from build123d import *

# Parameters (mm, degrees)
ESBO_O1_W                                            = 100
ESBO_O1_H                                            = 40
BASEPLATE_DEPTH                                      = 10
VERTBOSS_DEPTH                                       = 10
ESBO_O3_W                                            = 39.225392784
ESBO_O3_H                                            = 3
BOTTOMSLOT_DEPTH                                     = 121.933866224
REBAIXO_PARA_PARAFUSO_DE_CABE_A_SEXTAVAD_D           = 9
REBAIXO_PARA_PARAFUSO_DE_CABE_A_SEXTAVAD_CBORE_D     = 18.01
REBAIXO_PARA_PARAFUSO_DE_CABE_A_SEXTAVAD_CBORE_DEPTH = 5.68
FILETE1_R                                            = 8
FILETE2_R                                            = 3
FURO_DE_DI_METRO_7_0_7_2_D                           = 7


with BuildPart() as part:
    # Esboço1 → BasePlate (new body)
    with BuildSketch(Plane(origin=(0, 0, 0), x_dir=(1, 0, 0), z_dir=(0, 1, 0))):
        with Locations((50, 20)):
            Rectangle(ESBO_O1_W, ESBO_O1_H)
    extrude(amount=BASEPLATE_DEPTH)

    # Esboço2 → VertBoss (add)
    with BuildSketch(Plane.XY):
        with BuildLine():
            Line((30, 0), (30, 35))
            ThreePointArc((30, 35), (50, 55), (70, 35))
            Line((70, 35), (70, 0))
            Line((70, 0), (30, 0))
        make_face()
    extrude(amount=-VERTBOSS_DEPTH)

    # Esboço3 → BottomSlot (cut, through all)
    with BuildSketch(Plane.XY):
        with Locations((50, 1.5)):
            Rectangle(ESBO_O3_W, ESBO_O3_H)
    extrude(amount=-BOTTOMSLOT_DEPTH, mode=Mode.SUBTRACT)

    # Rebaixo para parafuso de cabeça sextavada de M81 (through all)
    with Locations(Plane.XY):
        with Locations((50, 35)):
            CounterBoreHole(REBAIXO_PARA_PARAFUSO_DE_CABE_A_SEXTAVAD_D / 2, REBAIXO_PARA_PARAFUSO_DE_CABE_A_SEXTAVAD_CBORE_D / 2, REBAIXO_PARA_PARAFUSO_DE_CABE_A_SEXTAVAD_CBORE_DEPTH)

    # Filete1
    # the kernel refuses this fillet: 8 mm, written as the material it adds along each edge
    with BuildSketch(Plane(origin=(69.612696392, 3, 0), x_dir=(-1, 0, 0), z_dir=(0, 0, -1))) as filete1_piece_1:
        with BuildLine():
            CenterArc((6.244997998, -8), FILETE1_R, 90, 51.317812547)
            Line((0, -3), (0, 0))
            Line((0, 0), (6.244997998, 0))
        make_face()
    extrude(amount=40)
    with BuildSketch(Plane(origin=(30.387303608, 3, 0), x_dir=(0, -1, 0), z_dir=(0, 0, -1))) as filete1_piece_2:
        with BuildLine():
            CenterArc((8, -6.244997998), FILETE1_R, 128.682187453, 51.317812547)
            Line((0, -6.244997998), (0, 0))
            Line((0, 0), (3, 0))
        make_face()
    extrude(amount=40)
    # the kernel refuses this fillet: 8 mm, written as the material it takes off along each edge
    with BuildSketch(Plane(origin=(0, -20, -40), x_dir=(0, 0, 1), z_dir=(0, 1, 0)), Plane(origin=(0, -20, 0), x_dir=(1, 0, 0), z_dir=(0, 1, 0))) as filete1_2_piece_1:
        with BuildLine():
            CenterArc((FILETE1_R, FILETE1_R), FILETE1_R, 180, 90)
            Line((0, FILETE1_R), (0, 0))
            Line((0, 0), (FILETE1_R, 0))
        make_face()
    extrude(amount=50, mode=Mode.SUBTRACT)
    with BuildSketch(Plane(origin=(100, -20, 0), x_dir=(-1, 0, 0), z_dir=(0, 1, 0)), Plane(origin=(100, -20, -40), x_dir=(0, 0, 1), z_dir=(0, 1, 0))) as filete1_2_piece_2:
        with BuildLine():
            CenterArc((FILETE1_R, -FILETE1_R), FILETE1_R, 90, 90)
            Line((0, -FILETE1_R), (0, 0))
            Line((0, 0), (FILETE1_R, 0))
        make_face()
    extrude(amount=50, mode=Mode.SUBTRACT)

    # Filete2
    filete2_edges = [part.edges().sort_by_distance(p)[0] for p in [
        (81, 10, 0),
        (30, 22.5, -10),
        (70, 22.5, -10),
        (30, 22.5, 0),
        (70, 22.5, 0),
        (50, 55, 0),
        (30, 10, -5),
        (50, 55, -10),
        (70, 10, -5),
        (50, 10, -10),
        (0, 10, -20),
        (50, 10, -40),
        (19, 10, 0),
        (100, 10, -20),
        (2.343145751, 10, -2.343145751),
        (97.656854249, 10, -37.656854249),
        (97.656854249, 10, -2.343145751),
        (2.343145751, 10, -37.656854249),
    ]]
    fillet(filete2_edges, radius=FILETE2_R)

    # Furo de diâmetro Ø7.0 (7)2 (through all)
    with Locations(Plane(origin=(0, 10, 0), x_dir=(1, 0, 0), z_dir=(0, 1, 0))):
        with Locations((11.205655488, 30.291277502), (89.117630716, 30.291277502)):
            Hole(FURO_DE_DI_METRO_7_0_7_2_D / 2)


solid = part.part
CAD build for the part. Positions are in the model's coordinates, mm. A direction names the side the tool comes from. Round coordinates to 2 decimals unless told otherwise and drop trailing zeros. Write each loop counter-clockwise with the first axis right and the second up, starting at its lowest first coordinate (ties: lowest second). Pieces come first, ordered by that corner, then holes.
(1) Drop flat-ended pins along their axis: P1, Ø6, axis at x = 77, z = -5.5, coming from the +Y side; P2, Ø5, axis at x = 35, y = 20, coming from the -Z side; P3, Ø3, axis at y = 28, z = -5.5, coming from the +X side. Give the stop position or say it passes through.
(2) Probe line 1 along Y through (x, z) = (50, -6.7); line 2 along Y through (x, z) = (50, -3) (3 decimals); line 3 along Y through (x, z) = (18.5, -30). List the from-to ranges inside material, lowest first.
(3) Mould opens along Y. For faces 1 (the face through (91.697, 4.93, -32.657)), 2 (the face through (54, 31, -5.68)), 3 (the face through (49.76, 10.86, -10.9)) say: pulls with the +Y half, pulls with the -Y half, needs draft (parallel to the pull), parting line crosses it, or undercut.
(4) 3-axis set-ups, long thin cutter, end or side, ignore diameter. For faces 4 (the face through (50, 28, -10)), 5 (the face through (69.1, 23.85, -0.86)), 6 (the face through (66.79, 2.23, -19.72)): which of +Z, -Z, +X, -X, +Y, -Y reach the whole face in a straight line?
(5) Slice it at B-B, the plane z = -19. Write the cut outline in (x, y).
(6) Slice it at C-C, the plane x = 25. Write the cut outline in (y, z), and give its area (3 significant figures).
(7) Slice it at A-A, the plane x = 50. Write the cut outline in (y, z) (3 decimals).
From the geometry:
1. P1: stops at y = 10
1. P2: stops at z = -10
1. P3: stops at x = 70
2. line 1: y = 3 to 30.5, 39.5 to 55
2. line 2: y = 3 to 25.995, 44.005 to 55
2. line 3: y = 0 to 10
3. face 1: needs draft
3. face 2: undercut
3. face 3: pulls with the +Y half
4. face 4: -Z, +X, -X, +Y
4. face 5: +Z, +X, +Y
4. face 6: +Z, -Z, -Y
5. outline: (0, 0) - (30.39, 0) arc R8 cw to (36.63, 3) - (63.37, 3) arc R8 cw to (69.61, 0) - (100, 0) - (100, 7) arc R3 ccw to (97, 10) - (3, 10) arc R3 ccw to (0, 7) - close
6. outline: (0, -40) - (7, -40) arc R3 ccw to (10, -37) - (10, -3) arc R3 ccw to (7, 0) - (0, 0) - close
6. area: 396 mm2
7. outline: (3, -40) - (7, -40) arc R3 ccw to (10, -37) - (10, -13) arc R3 cw to (13, -10) - (30.5, -10) - (30.5, -5.68) - (25.995, -5.68) - (25.995, 0) - (3, 0) - close; (39.5, -10) - (52, -10) arc R3 ccw to (55, -7) - (55, -3) arc R3 ccw to (52, 0) - (44.005, 0) - (44.005, -5.68) - (39.5, -5.68) - close
